Input: part model. Units: mm. Frame: model coordinates. A direction names the side the tool comes from. Give positions to 0.01 mm unless a question says otherwise; leave off trailing zeros. Loops run counter-clockwise (first coordinate to the right, second up) from the corner with the lowest first, then second, coordinate; pieces in that order, holes last. Notation, with made-up numbers: M -38.5,61 L 18.5,61 A22 cw 18.5,71 Z; hole C -18.75,-1.5 d11. An arc over 180 degrees is marked long. One line per item, written item: value. Start each with the question number.
(1) Pull-direction query (X, two-part tool) for faces 4 (the cylindrical face through (23.846, -6.423, 7.509)), 5 (the flat face through (0, -37, 0)), 6 (the cylindrical face through (11.73, -5.92, 13.08)); classes: released by +X, released by -X, zero draft, split by the parting line, or undercut.
(2) Access query for faces 1 (the cylindrical face through (11.923, -24.325, 3.755)), 2 (the cylindrical face through (-12.27, -5.92, 13.08)), 3 (the flat face through (5, 0, -5)). Directions: +Z, -Z, +X, -X, +Y, -Y. A direction counts if a zero-diameter tool reaches every point of the face in a straight line with its end or side. Return the directions, or none.
(3) Pin query (flat end, axial travel): P1, Ø10, axis at y = -33, z = -0.5, coming from the -X side; P2, Ø4, axis at x = 12, z = 14.3, coming from the +Y side; P3, Ø5, axis at y = -10.5, z = -9, coming from the +X side. Return the tip coordinate at first contact, or that it passes through.
(4) Section C-C on y = -5. Output: boundary loops of the cut face in (x, z).
(5) Section A-A on x = 0. Output: boundary loops of the cut face in (y, z), plus the area to 3 significant figures.
(6) Section D-D on y = -28.5. Output: boundary loops of the cut face in (x, z).
(7) Ray query, line 1 along Y through (x, z) = (8, -11); line 2 along Y through (x, z) = (8, -6); line 3 along Z through (x, y) = (-13, -9). Return the intervals inside material, ascending. Write a range as from..to.
(8) Section B-B on z = 0. Output: boundary loops of the cut face in (x, y), plus the area to 3 significant figures.
```python
from build123d import *

# Parameters (mm, degrees)
F0_R     = 6
F1_DEPTH = 3
F0_R_2   = 12.5
F2_DEPTH = 37
F0_R_3   = 25
F0_R_4   = 1.25
F3_DEPTH = 12
F4_DEPTH = 37
F5_SIZE  = 1


with BuildPart() as f1:
    # F0 (on Front) → F1 (new body)
    with BuildSketch(Plane.XZ):
        Circle(F0_R)
    extrude(amount=-F1_DEPTH)



with BuildPart() as f2:
    # F0 (on Front) → F2 (new body)
    with BuildSketch(Plane.XZ):
        Circle(F0_R_2)
        Circle(F0_R, mode=Mode.SUBTRACT)
    extrude(amount=F2_DEPTH)

    # F0 (on Front) → F3 (join)
    with BuildSketch(Plane.XZ):
        Circle(F0_R_3)
        with Locations((-12.000845, 14.30205)):
            Circle(F0_R_4, mode=Mode.SUBTRACT)
        Circle(F0_R_2, mode=Mode.SUBTRACT)
        with Locations((0, 18.67)):
            Circle(F0_R_4, mode=Mode.SUBTRACT)
        with Locations((12.000845, 14.30205)):
            Circle(F0_R_4, mode=Mode.SUBTRACT)
    extrude(amount=F3_DEPTH)


with BuildPart() as f1_1:
    add(f1.part)

    add(f2.part)  # F4 merges F2
    # F0 (on Front) → F4 (join)
    with BuildSketch(Plane.XZ):
        Circle(F0_R)
    extrude(amount=F4_DEPTH)

    # F5
    f5_edges = [f1_1.edges().sort_by_distance(p)[0] for p in [
        (-25, 0, 0),
        (-6, 3, 0),
    ]]
    chamfer(f5_edges, length=F5_SIZE)


solid = f1_1.part
```
Output values:
1. face 4: split by the parting line
1. face 5: zero draft
1. face 6: undercut
2. face 1: -Y
2. face 2: +Y, -Y
2. face 3: +Y
3. P1: stops at x = -12.5
3. P2: stops at y = 0
3. P3: stops at x = 24.14
4. outline: C 0,0 d50; hole C -12,14.3 d2.5; hole C 0,18.67 d2.5; hole C 12,14.3 d2.5
5. outline: M -37,-12.5 L -12,-12.5 L -12,-25 L -1,-25 L 0,-24 L 0,-6 L 2,-6 L 3,-5 L 3,5 L 2,6 L 0,6 L 0,17.42 L -12,17.42 L -12,12.5 L -37,12.5 Z; M -12,19.92 L 0,19.92 L 0,24 L -1,25 L -12,25 Z
5. area: 1,230 mm²
6. outline: C 0,0 d25
7. line 1: y = -12..0
7. line 2: y = -37..0
7. line 3: z = -21.35..13.55, 15.05..21.35
8. outline: M -25,-12 L -12.5,-12 L -12.5,-37 L 12.5,-37 L 12.5,-12 L 25,-12 L 25,-1 L 24,0 L 6,0 L 6,2 L 5,3 L -5,3 L -6,2 L -6,0 L -24,0 L -25,-1 Z
8. area: 1,260 mm²
